from build123d import *

# Parameters (mm, degrees)
SKICA1_W                 = 200
SKICA1_H                 = 100
P_IDAT_VYSUNUT_M1_DEPTH  = 20
P_IDAT_VYSUNUT_M2_DEPTH  = 50
ODEBRAT_VYSUNUT_M1_REACH = 236.307
SKICA4_R                 = 50
SKICA7_R                 = 7.5
P_IDAT_VYSUNUT_M3_DEPTH  = 50


with BuildPart() as part:
    # Skica1 → Přidat vysunutím1 (new body)
    with BuildSketch(Plane.XY):
        with Locations((100, 50)):
            Rectangle(SKICA1_W, SKICA1_H)
    extrude(amount=P_IDAT_VYSUNUT_M1_DEPTH)

    # Skica2 → Přidat vysunutím2 (add)
    with BuildSketch(Plane.XY.offset(20)):
        Polygon((120, 0), (160, 0), (160, 100), (155, 100), (155, 70), (130, 70), (130, 100), (120, 100), align=None)
    extrude(amount=P_IDAT_VYSUNUT_M2_DEPTH)

    # Odebrat vysunutím1: up to this face of the body (flat: up to its plane)
    odebrat_vysunut_m1_end = Plane(part.part.faces().sort_by_distance((139.423076923, 41.923076923, 70))[0])
    # Skica4 → Odebrat vysunutím1 (cut, up to the picked face)
    with BuildSketch(Plane(origin=(0, 0, 0), x_dir=(-1, 0, 0), z_dir=(0, 0, -1)), mode=Mode.PRIVATE) as odebrat_vysunut_m1_sk1:
        with Locations((-80, 0)):
            Circle(SKICA4_R)
    odebrat_vysunut_m1_tool1 = split(extrude(odebrat_vysunut_m1_sk1.sketch, amount=-ODEBRAT_VYSUNUT_M1_REACH, mode=Mode.PRIVATE), bisect_by=odebrat_vysunut_m1_end, keep=Keep.BOTH, mode=Mode.PRIVATE)
    add(odebrat_vysunut_m1_tool1.solids().sort_by(Axis((80, 0, 0), (0, 0, 1)))[0], mode=Mode.SUBTRACT)

    # Skica7 → Přidat vysunutím3 (add)
    with BuildSketch(Plane.XY.offset(20)):
        with Locations(Location((12, 80, 0), (0, 0, 180))):
            Circle(SKICA7_R)
    extrude(amount=P_IDAT_VYSUNUT_M3_DEPTH)


solid = part.part
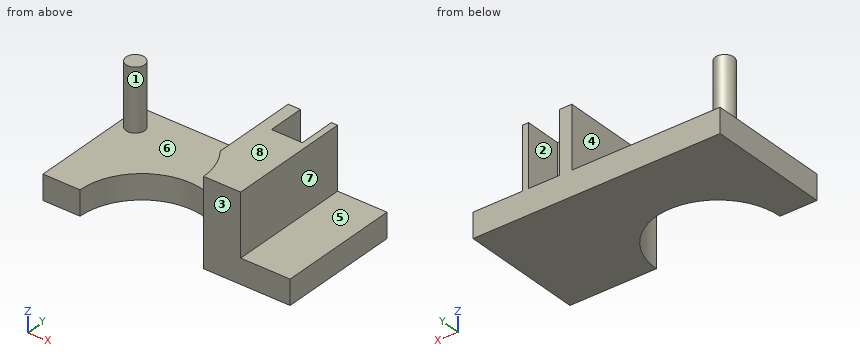
For this review, take the finished solid that the model builds, in its own axes (mm). Face numbers are marked on the shaded views. A direction names the side the tool comes from. Round coordinates to 2 decimals unless told otherwise and drop trailing zeros. Write each loop counter-clockwise with the first axis right and the second up, starting at its lowest first coordinate (ties: lowest second). Pieces come first, ordered by that corner, then holes. Notation, with made-up numbers: (-10, -5) - (13, -5) arc R32 ccw to (13, 28) - close; hole circle Ø8 at (16, 16). An arc over 180 degrees is marked (long way). Use a Markdown table: item, result.
Q1. Machinability: for the marked faces 1, 2, 3, 4 and 5, which of the approach directions +Z, -Z, +X, -X, +Y, -Y give a long, thin tool a straight path to every point of the face, cutting with its end or side? Answer none if there is none.
Derived:
| item | result |
|---|---|
| face 1 | +Z |
| face 2 | +Z, +Y |
| face 3 | +Z, -Z, +X, -X, -Y |
| face 4 | +Z, +Y, -Y |
| face 5 | +Z, +X, +Y, -Y |
Q2. Wall thickness on line 1 along X through (y, z) = (93, 42.5); line 2 along X through (y, z) = (82, 30); line 3 along X through (y, z) = (38.5, 67): over which ranges is each line inside the solid? List them lowest first.
Derived:
| item | result |
|---|---|
| line 1 | x = 120 to 130, 155 to 160 |
| line 2 | x = 4.77 to 19.23, 120 to 130, 155 to 160 |
| line 3 | x = 120 to 160 |
Q3. We need section C-C (y = 80). Give the boundary of the cut face in (x, z).
Derived:
| item | result |
|---|---|
| outline | (0, 0) - (200, 0) - (200, 20) - (160, 20) - (160, 70) - (155, 70) - (155, 20) - (130, 20) - (130, 70) - (120, 70) - (120, 20) - (19.5, 20) - (19.5, 70) - (4.5, 70) - (4.5, 20) - (0, 20) - close |
Q4. The part is to be moulded in two halves that separate along X. For the marked faces 6, 7 and 8, say which applies: pulls with the +X half, pulls with the -X half, needs draft (parallel to the pull), parting line crosses it, or undercut.
Derived:
| item | result |
|---|---|
| face 6 | undercut |
| face 7 | pulls with the +X half |
| face 8 | needs draft |
Q5. We need section B-B (x = 12). Give the boundary of the cut face in (y, z), plus the area to 3 significant figures.
Derived:
| item | result |
|---|---|
| outline | (0, 0) - (100, 0) - (100, 20) - (87.5, 20) - (87.5, 70) - (72.5, 70) - (72.5, 20) - (0, 20) - close |
| area | 2,750 mm2 |
Q6. We need section A-A (z = 27). Give the boundary of the cut face in (x, y), plus the area to 3 significant figures.
Derived:
| item | result |
|---|---|
| outline | circle Ø15 at (12, 80); (120, 30) arc R50 cw to (130, 0) - (160, 0) - (160, 100) - (155, 100) - (155, 70) - (130, 70) - (130, 100) - (120, 100) - close |
| area | 3,220 mm2 |
Q7. Clearance check with flat-ended pins moving along their axes: pin 1 (9 mm diameter, centred on y = 85, z = 49.5, fed in from -X); pin 2 (15 mm diameter, centred on y = 50, z = 55, fed in from +X); pin 3 (2 mm diameter, centred on y = 60.5, z = 36, fed in from -X). State where each tip first meets the part, or that it passes through.
Derived:
| item | result |
|---|---|
| pin 1 | stops at x = 4.52 |
| pin 2 | stops at x = 160 |
| pin 3 | stops at x = 120 |
Q8. We need section D-D (y = 47.5). Give the boundary of the cut face in (x, z), plus the area to 3 significant figures.
Derived:
| item | result |
|---|---|
| outline | (0, 0) - (64.39, 0) - (64.39, 20) - (0, 20) - close; (95.61, 0) - (200, 0) - (200, 20) - (160, 20) - (160, 70) - (120, 70) - (120, 20) - (95.61, 20) - close |
| area | 5,380 mm2 |
